```python
from build123d import *

# Parameters (mm, degrees)
BOSS_EXTRUDE1_DEPTH = 295
SKETCH2_R           = 1.75
CUT_EXTRUDE1_DEPTH  = 296.105913191
SKETCH2_3_R         = 3
SKETCH2_3_R_2       = 1.75
CUT_EXTRUDE2_DEPTH  = 3.5
LPATTERN1_COUNT     = 15
LPATTERN1_PITCH     = 20
SKETCH4_R           = 4.15
BOSS_EXTRUDE2_DEPTH = 2.25
LPATTERN2_COUNT     = 2
LPATTERN2_PITCH     = 280


with BuildPart() as part:
    # Sketch1 → Boss-Extrude1 (new body)
    with BuildSketch(Plane.XY):
        Polygon((4.5, 0), (-4.5, 0), (-4.5, 3), (-3.775867518, 3.607619299), (-3.168844988, 3.607619299), (-3.168844988, 4.95), (-3.775867518, 4.95), (-4.5, 5.557619299), (-4.5, 6.5), (0, 6.5), (4.5, 6.5), (4.5, 5.557619299), (3.775867518, 4.95), (3.168844988, 4.95), (3.168844988, 3.607619299), (3.775867518, 3.607619299), (4.5, 3), align=None)
    extrude(amount=BOSS_EXTRUDE1_DEPTH)

    # Sketch2 → Cut-Extrude1 (cut, through all)
    with BuildSketch(Plane(origin=(0, 6.5, 0), x_dir=(1, 0, 0), z_dir=(0, 1, 0))):
        with Locations(Location((0, -7.5, 0), (0, 0, 180))):
            Circle(SKETCH2_R)
    cut_extrude1 = extrude(amount=-CUT_EXTRUDE1_DEPTH, mode=Mode.SUBTRACT)

    # Sketch2_3 → Cut-Extrude2 (cut)
    with BuildSketch(Plane(origin=(0, 6.5, 0), x_dir=(1, 0, 0), z_dir=(0, 1, 0))):
        with Locations(Location((0, -7.5, 0), (0, 0, 180))):
            Circle(SKETCH2_3_R)
        with Locations(Location((0, -7.5, 0), (0, 0, 180))):
            Circle(SKETCH2_3_R_2, mode=Mode.SUBTRACT)
    cut_extrude2 = extrude(amount=-CUT_EXTRUDE2_DEPTH, mode=Mode.SUBTRACT)

    # LPattern1: Cut-Extrude1, Cut-Extrude2 ×15
    with Locations(*[(0, 0, i * LPATTERN1_PITCH) for i in range(1, LPATTERN1_COUNT)]):
        add(cut_extrude1, mode=Mode.SUBTRACT)
        add(cut_extrude2, mode=Mode.SUBTRACT)

    # Sketch4 → Boss-Extrude2 (add)
    with BuildSketch(Plane(origin=(0, 6.5, 0), x_dir=(1, 0, 0), z_dir=(0, 1, 0))):
        with Locations(Location((0, -7.5, 0), (0, 0, 90))):
            Circle(SKETCH4_R)
    boss_extrude2 = extrude(amount=BOSS_EXTRUDE2_DEPTH)

    # LPattern2: Boss-Extrude2 ×2
    with Locations(*[(0, 0, i * LPATTERN2_PITCH) for i in range(1, LPATTERN2_COUNT)]):
        add(boss_extrude2)


solid = part.part
```
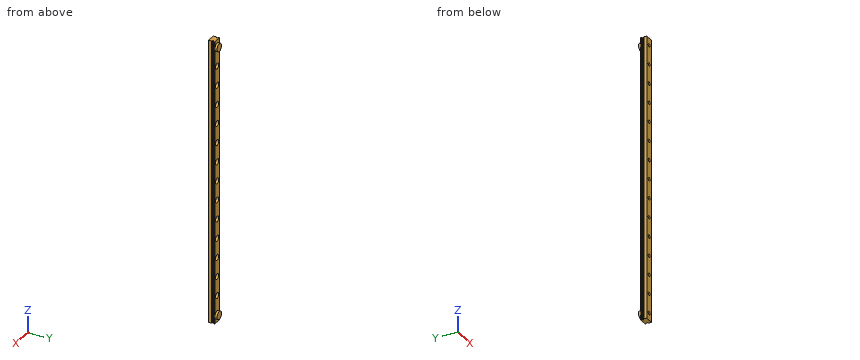
Work out the finished part from the listing and answer in its coordinate system (mm). Give positions to 0.01 mm unless a question says otherwise; leave off trailing zeros. Write each loop counter-clockwise with the first axis right and the second up, starting at its lowest first coordinate (ties: lowest second). Pieces come first, ordered by that corner, then holes. Notation, with made-up numbers: (-1, 32.25) - (57, 32.25) arc R21 ccw to (57, 61.25) - close; hole circle Ø5 at (22.25, 40). An arc over 180 degrees is marked (long way). Use one line per item in the form item = value.
1. Consider L1, parallel to X at y = 1.15, z = 187.5; L2, parallel to Y at x = 0.5, z = 38.5; L3, parallel to X at y = 3.7, z = 107.5. Determine where each line is inside the solid, lowest interval first.
Filled in:
L1 = -4.5 to -1.75, 1.75 to 4.5
L2 = 0 to 6.5
L3 = -3.17 to -3, 3 to 3.17
2. A cutting plane is placed at A-A (z = 36.5). Write down the section's boundary in (x, y), and give its area (3 significant figures).
Filled in:
outline = (-4.5, 0) - (4.5, 0) - (4.5, 3) - (3.78, 3.61) - (3.17, 3.61) - (3.17, 4.95) - (3.78, 4.95) - (4.5, 5.56) - (4.5, 6.5) - (-4.5, 6.5) - (-4.5, 5.56) - (-3.78, 4.95) - (-3.17, 4.95) - (-3.17, 3.61) - (-3.78, 3.61) - (-4.5, 3) - close
area = 54.0 mm^2
3. Each of these flat-tipped pins is pushed along its axis until it touches: pin 1 Ø0.5 at (x, z) = (-3.5, 174.5) entering from +Y; pin 2 Ø4 at (x, z) = (0, 7.5) entering from -Y; pin 3 Ø4.5 at (x, z) = (0, 27.5) entering from +Y. Where does it stop, or does it pass through?
Filled in:
pin_1 = 6.5
pin_2 = 0
pin_3 = 3
